Geometry: final body of the model. Coordinates: model frame, mm. A direction names the side the tool comes from. Give positions to 0.01 mm unless a question says otherwise; leave off trailing zeros. Order: outer loops, then holes, each group sorted by start corner. A loop starts at its lowest first (then second) coordinate and runs counter-clockwise, first axis right, second up. Notation, with made-up numbers: (34, 71.5) -> (82, 71.5) arc R27 ccw to (82, 87.5) -> close; hole circle Ø5 at (-26.75, 21). An arc over 180 degrees is marked (long way). Write item = value, one per line.
```python
from build123d import *

# Parameters (mm, degrees)
F1_DEPTH = 1.778
F3_DEPTH = 10.16
F4_W     = 16.85848
F4_H     = 4.34721
F5_DEPTH = 1.27


with BuildPart() as f1:
    # F0 (on Top) → F1 (new body)
    with BuildSketch(Plane.XY):
        with BuildLine():
            Line((0, 27.3558), (0, 0))
            Line((0, 0), (46.800594, 9.0932))
            ThreePointArc((46.800594, 9.0932), (26.687452, 44.698298), (-10.16, 62.4332))
            Line((-10.16, 62.4332), (-10.16, 47.6758))
            Line((-10.16, 47.6758), (0, 47.6758))
            Line((0, 47.6758), (0, 33.7058))
            Line((0, 33.7058), (-2.54, 33.7058))
            Line((-2.54, 33.7058), (-2.54, 36.2458))
            Line((-2.54, 36.2458), (-7.62, 36.2458))
            Line((-7.62, 36.2458), (-7.62, 27.3558))
            Line((-7.62, 27.3558), (0, 27.3558))
        make_face()
    extrude(amount=F1_DEPTH)

    # F2 (on face) → F3 (join)
    with BuildSketch(Plane.XY.offset(1.778)):
        Polygon((2.986613, 6.865549), (0, 0), (46.800594, 9.0932), (43.356929, 14.709367), align=None)
    extrude(amount=F3_DEPTH)

    # F4 (on face) → F5 (join)
    with BuildSketch(Plane.XY.offset(1.778)):
        with Locations((0.80924, 29.529405)):
            Rectangle(F4_W, F4_H)
    extrude(amount=F5_DEPTH)


solid = f1.part
```
1) Mould query, pull axis Y, two halves, no side actions, for faces 1 (the face through (27.11, 44.3, 0.88)), 2 (the face through (18, 32, 0)), 3 (the face through (-5, 47.676, 1)). Classes: +Y half, -Y half, draft (parallel to the pull), parting line (faces both ways), or undercut.
Check sheet entries:
face_1 = +Y half
face_2 = draft
face_3 = undercut
2) Section query B-B (y = 11.5). Output: boundary loops of the cut face in (x, z).
Check sheet entries:
outline = (0, 0) -> (46.24, 0) -> (46.24, 1.78) -> (45.32, 1.78) -> (45.32, 11.94) -> (26.84, 11.94) -> (26.84, 1.78) -> (0, 1.78) -> close
3) Section query A-A (x = -3.5). Output: boundary loops of the cut face in (y, z).
Check sheet entries:
outline = (27.36, 0) -> (36.25, 0) -> (36.25, 1.78) -> (31.7, 1.78) -> (31.7, 3.05) -> (27.36, 3.05) -> close; (47.68, 0) -> (61.12, 0) -> (61.12, 1.78) -> (47.68, 1.78) -> close
4) Section query D-D (z = 5.5). Output: boundary loops of the cut face in (x, y).
Check sheet entries:
outline = (0, 0) -> (46.8, 9.09) -> (43.36, 14.71) -> (2.99, 6.87) -> close
5) First-contact query: P1, Ø0.5, axis at x = -6, z = 1, coming from the +Y side; P2, Ø0.5, axis at y = 35, z = 1, coming from the +X side; P3, Ø2, axis at x = -1, z = 1, coming from the +Y side; P4, Ø5, axis at x = 34, y = 26.5, coming from the -Z side. Flat tips, straight axial feed; report the tip coordinate or a pass-through.
Check sheet entries:
P1 = 61.75
P2 = 35.43
P3 = 60.73
P4 = 0
6) Section query C-C (x = 15.5). Output: boundary loops of the cut face in (y, z).
Check sheet entries:
outline = (3.01, 0) -> (53.2, 0) -> (53.2, 1.78) -> (9.3, 1.78) -> (9.3, 11.94) -> (3.01, 11.94) -> close
7) Reachability of faces 4 (the face through (-1, 27.356, 2)), 5 (the face through (-1, 33.706, 1)), 6 (the face through (-5, 36.246, 1)), 7 (the face through (-7.62, 31, 1)) from +Z, -Z, +X, -X, +Y, -Y: full face, straight path, thin tool, end or side. Return the list, or none.
Check sheet entries:
face_4 = +Z, -X
face_5 = +Z, -Z
face_6 = +Z, -Z, -X
face_7 = +Z, -Z, -X, -Y
8) Line query: line 1 (Z direction, x = 4.5, y = 24.5); line 2 (Y direction, x = 23.5, z = 2); line 3 (Y direction, x = 25.5, z = 7.5). Output: solid intervals per line, ascending. Write a range as from..to.
Check sheet entries:
line_1 = 0..1.78
line_2 = 4.57..10.85
line_3 = 4.95..11.24
